The drawing under review shows one solid part. Ordinate dimensions are in mm from its lowest x, y, z. Coordinates: 2 decimals unless noted, no trailing zeros. Order: outer loops, then holes, each group sorted by start corner. A loop starts at its lowest first (then second) coordinate and runs counter-clockwise, first axis right, second up. Notation, with made-up numbers: (82, -17) -> (101, -17) arc R23 ccw to (101, 8) -> close; hole circle Ø2 at (-23.5, 14.5). An arc over 180 degrees is marked (long way). Use a Markdown table: item, result. Add a question column.
Q1. Wall thickness on probe 1 along X at (y, z) = (29, 170); probe 2 along Z at (x, y) = (185.5, 10.5): over which ranges is each line inside the solid? List them lowest first.
Q2. The part is to be moulded in two halves that separate along Z. For the marked faces 1 and 2, say which applies: pulls with the +Z half, pulls with the -Z half, needs draft (parallel to the pull), parting line crosses it, or undercut.
Q3. Add section C-C (y = 33.5). State the section outline as (x, z) points.
Q4. Add section A-A (z = 170). State the section outline as (x, y) points.
Q5. Add section B-B (x = 170). State the section outline as (y, z) points, then the cut area to 3 significant figures.
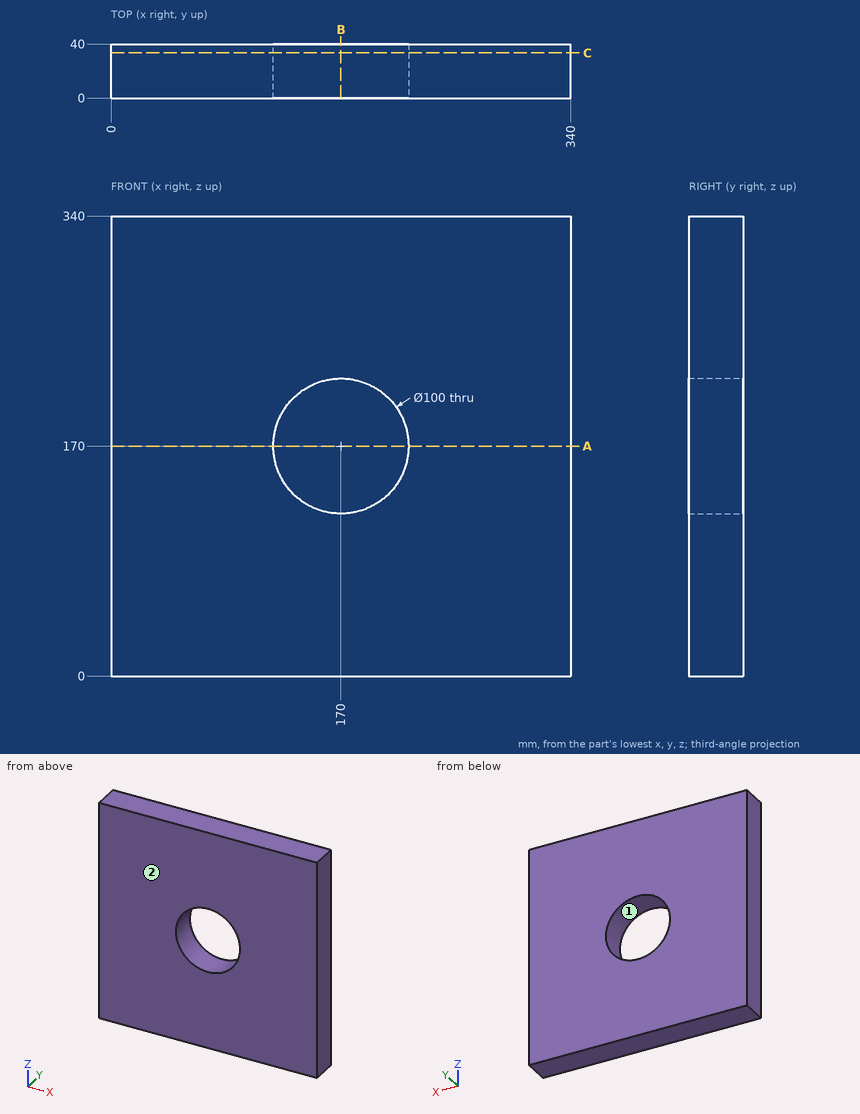
Established:
| question | item | result |
|---|---|---|
| 1 | probe 1 | 0 to 120, 220 to 340 |
| 1 | probe 2 | 0 to 122.46, 217.54 to 340 |
| 2 | face 1 | undercut |
| 2 | face 2 | needs draft |
| 3 | outline | (0, 0) -> (340, 0) -> (340, 340) -> (0, 340) -> close; hole circle Ø100 at (170, 170) |
| 4 | outline | (0, 0) -> (120, 0) -> (120, 40) -> (0, 40) -> close; (220, 0) -> (340, 0) -> (340, 40) -> (220, 40) -> close |
| 5 | outline | (0, 0) -> (40, 0) -> (40, 120) -> (0, 120) -> close; (0, 220) -> (40, 220) -> (40, 340) -> (0, 340) -> close |
| 5 | area | 9,600 mm^2 |
